For this review, use the dimensioned drawing (mm, ordinates from the lowest corner) and the shaded views. A direction names the side the tool comes from. Round coordinates to 2 decimals unless told otherwise and drop trailing zeros. Order: outer loops, then holes, each group sorted by start corner. A loop starts at its lowest first (then second) coordinate and runs counter-clockwise, first axis right, second up. Notation, with made-up numbers: (0.25, -3) - (20.25, -3) arc R22 ccw to (20.25, 22) - close; hole circle Ø10 at (14.5, -19.75). An arc over 180 degrees is marked (long way). Write item = value, one per line.
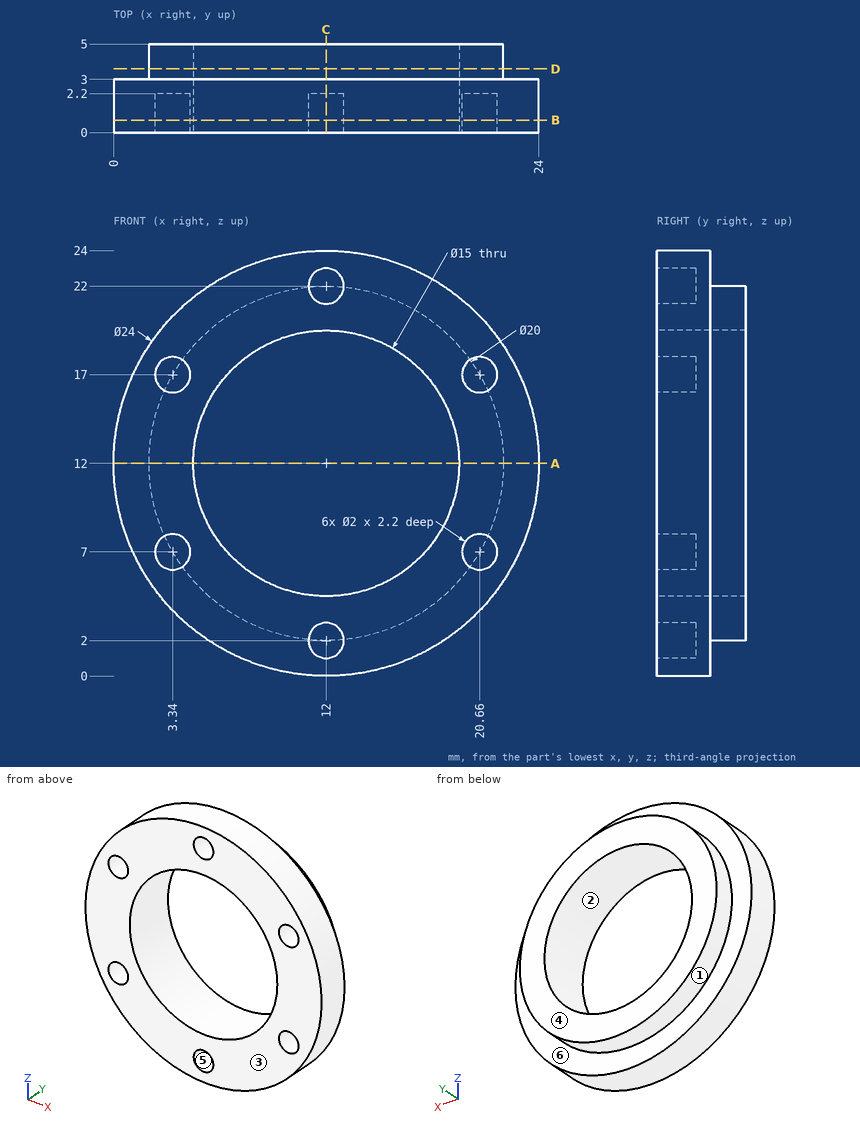
Item 1: Take a section at B-B, the plane y = 0.7. State the section outline as (x, z) points.
Data:
outline = circle Ø24 at (12, 12); hole circle Ø2 at (3.34, 7); hole circle Ø2 at (3.34, 17); hole circle Ø15 at (12, 12); hole circle Ø2 at (12, 2); hole circle Ø2 at (12, 22); hole circle Ø2 at (20.66, 7); hole circle Ø2 at (20.66, 17)
Item 2: For the marked faces 4, 5 and 6, list the 3-axis set-ups (+Z, -Z, +X, -X, +Y, -Y) from which the entire face can be reached by the end or side of a thin tool; tool diameter is ignored.
Data:
face_4 = +Z, -Z, +X, -X, +Y
face_5 = -Y
face_6 = +Y
Item 3: Take a section at D-D, the plane y = 3.6. State the section outline as (x, z) points.
Data:
outline = circle Ø20 at (12, 12); hole circle Ø15 at (12, 12)
Item 4: Insertion check: P1, Ø13.5, axis at x = 12, z = 12, coming from the +Y side; P2, Ø1, axis at x = 3, z = 17, coming from the -Y side; P3, Ø1, axis at y = 2, z = 4.5, coming from the -X side; P4, Ø1.5, axis at x = 13.5, y = 2, coming from the -Z side. Each pin has a flat end and moves straight along its axis. Give the tip position at first contact, or say it passes through.
Data:
P1 = through
P2 = 2.2
P3 = 2.25
P4 = 0.02
Item 5: Take a section at C-C, the plane x = 12. State the section outline as (y, z) points, and give its area (3 significant figures).
Data:
outline = (0, 0) - (3, 0) - (3, 2) - (5, 2) - (5, 4.5) - (0, 4.5) - (0, 3) - (2.2, 3) - (2.2, 1) - (0, 1) - close; (0, 19.5) - (5, 19.5) - (5, 22) - (3, 22) - (3, 24) - (0, 24) - (0, 23) - (2.2, 23) - (2.2, 21) - (0, 21) - close
area = 28.2 mm2
Item 6: For line 1 along Z through (x, y) = (12, 1.25); line 2 along Z through (x, y) = (3.5, 1.8); line 3 along Y through (x, z) = (3.75, 17.5), list the stretches that pass through material, from the lowest coordinate up. Write a range as [from, to].
Data:
line_1 = [0, 1], [3, 4.5], [19.5, 21], [23, 24]
line_2 = [3.53, 6.01], [7.99, 16.01], [17.99, 20.47]
line_3 = [2.2, 5]
Item 7: The part is to be moulded in two halves that separate along Z. For the marked faces 1, 2 and 3, say which applies: +Z half, -Z half, draft (parallel to the pull), parting line (faces both ways), or undercut.
Data:
face_1 = parting line
face_2 = undercut
face_3 = draft
Item 8: Take a section at A-A, the plane z = 12. State the section outline as (x, y) points, and give its area (3 significant figures).
Data:
outline = (0, 0) - (4.5, 0) - (4.5, 5) - (2, 5) - (2, 3) - (0, 3) - close; (19.5, 0) - (24, 0) - (24, 3) - (22, 3) - (22, 5) - (19.5, 5) - close
area = 37.0 mm2
